CAD build for the part. Positions are in the model's coordinates, mm. Coordinates: 2 decimals unless noted, no trailing zeros. Loops run counter-clockwise (first coordinate to the right, second up) from the corner with the lowest first, then second, coordinate; pieces in that order, holes last.
1) Saw through at B-B, the plane x = 95. Write the cut outline in (y, z), and give its area (3 significant figures).
2) Saw through at A-A, the plane y = 9. Write the cut outline in (x, z).
3) Wall check: line 1 along Y through (x, z) = (95, 75.05); line 2 along X through (y, z) = (9, 73.75); line 3 along Y through (x, z) = (99.5, 74.9). Give the ranges that are in metal, low to high.
```python
from build123d import *

# Parameters (mm, degrees)
CYLINDER015_R     = 1.6
CYLINDER015_DEPTH = 22
CYLINDER016_R     = 1.6
CYLINDER016_DEPTH = 22
CYLINDER013_R     = 1.6
CYLINDER013_DEPTH = 22
CYLINDER014_R     = 1.6
CYLINDER014_DEPTH = 22
BOX006_W          = 105
BOX006_H          = 150
BOX006_DEPTH      = 3
FILLET004_R       = 15


with BuildPart() as cilindro015:
    # Cylinder015 → Cylinder015 (new body)
    with BuildSketch(Plane(origin=(10, 141, 51), x_dir=(1, 0, 0), z_dir=(0, 0, 1))):
        Circle(CYLINDER015_R)
    extrude(amount=CYLINDER015_DEPTH)


with BuildPart() as cilindro016:
    # Cylinder016 → Cylinder016 (new body)
    with BuildSketch(Plane(origin=(95, 141, 51), x_dir=(1, 0, 0), z_dir=(0, 0, 1))):
        Circle(CYLINDER016_R)
    extrude(amount=CYLINDER016_DEPTH)


with BuildPart() as cilindro013:
    # Cylinder013 → Cylinder013 (new body)
    with BuildSketch(Plane(origin=(95, 9, 51), x_dir=(1, 0, 0), z_dir=(0, 0, 1))):
        Circle(CYLINDER013_R)
    extrude(amount=CYLINDER013_DEPTH)


with BuildPart() as fusion006:
    # Cylinder014 → Cylinder014 (new body)
    with BuildSketch(Plane(origin=(10, 9, 51), x_dir=(1, 0, 0), z_dir=(0, 0, 1))):
        Circle(CYLINDER014_R)
    extrude(amount=CYLINDER014_DEPTH)

    # Fusion006: union Cilindro015, Cilindro016, Cilindro013
    add(cilindro015.part)
    add(cilindro016.part)
    add(cilindro013.part)


with BuildPart() as fusion006_1:
    # Fusion006 placement: moved
    add(fusion006.part.moved(Location((0, 0, 7))))


with BuildPart() as cut008:
    # Box006 → Box006 (new body)
    with BuildSketch(Plane.XY):
        with Locations((52.5, 75)):
            Rectangle(BOX006_W, BOX006_H)
    extrude(amount=BOX006_DEPTH)

    # Fillet004
    fillet004_edges = [cut008.edges().sort_by_distance(p)[0] for p in [
        (0, 0, 1.5),
        (0, 150, 1.5),
        (105, 0, 1.5),
        (105, 150, 1.5),
    ]]
    fillet(fillet004_edges, radius=FILLET004_R)


with BuildPart() as cut008_1:
    # Fillet004 placement: moved
    add(cut008.part.moved(Location((0, 0, 72))))

    # Cut008: cut Fusion006
    add(fusion006_1.part, mode=Mode.SUBTRACT)


with BuildPart() as cut008_2:
    # Cut008 placement: moved
    add(cut008_1.part.moved(Location((0, 0, 1))))


solid = cut008_2.part
```
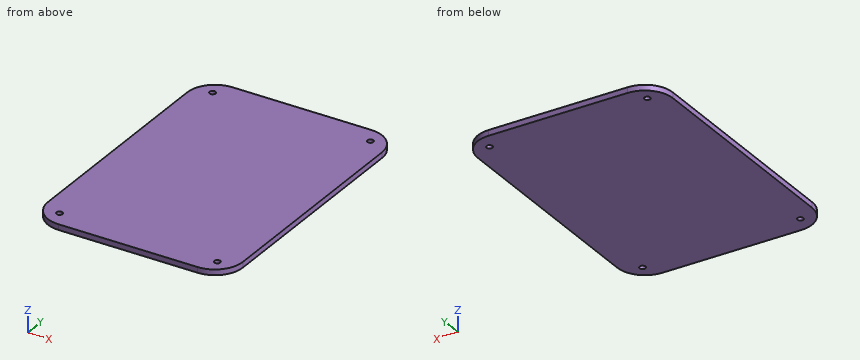
Data:
1. outline: (0.86, 73) - (7.4, 73) - (7.4, 76) - (0.86, 76) - close; (10.6, 73) - (139.4, 73) - (139.4, 76) - (10.6, 76) - close; (142.6, 73) - (149.14, 73) - (149.14, 76) - (142.6, 76) - close
1. area: 426 mm2
2. outline: (1.25, 73) - (8.4, 73) - (8.4, 76) - (1.25, 76) - close; (11.6, 73) - (93.4, 73) - (93.4, 76) - (11.6, 76) - close; (96.6, 73) - (103.75, 73) - (103.75, 76) - (96.6, 76) - close
3. line 1: y = 0.86 to 7.4, 10.6 to 139.4, 142.6 to 149.14
3. line 2: x = 1.25 to 8.4, 11.6 to 93.4, 96.6 to 103.75
3. line 3: y = 3.39 to 146.61
